Input: dimensioned drawing with shaded views. Units: mm. Origin: part minimum x, y, z. Give positions to 0.01 mm unless a question says otherwise; leave off trailing zeros. Write each loop counter-clockwise with the first axis right and the second up, starting at its lowest first coordinate (ties: lowest second). Pieces come first, ordered by that corner, then holes.
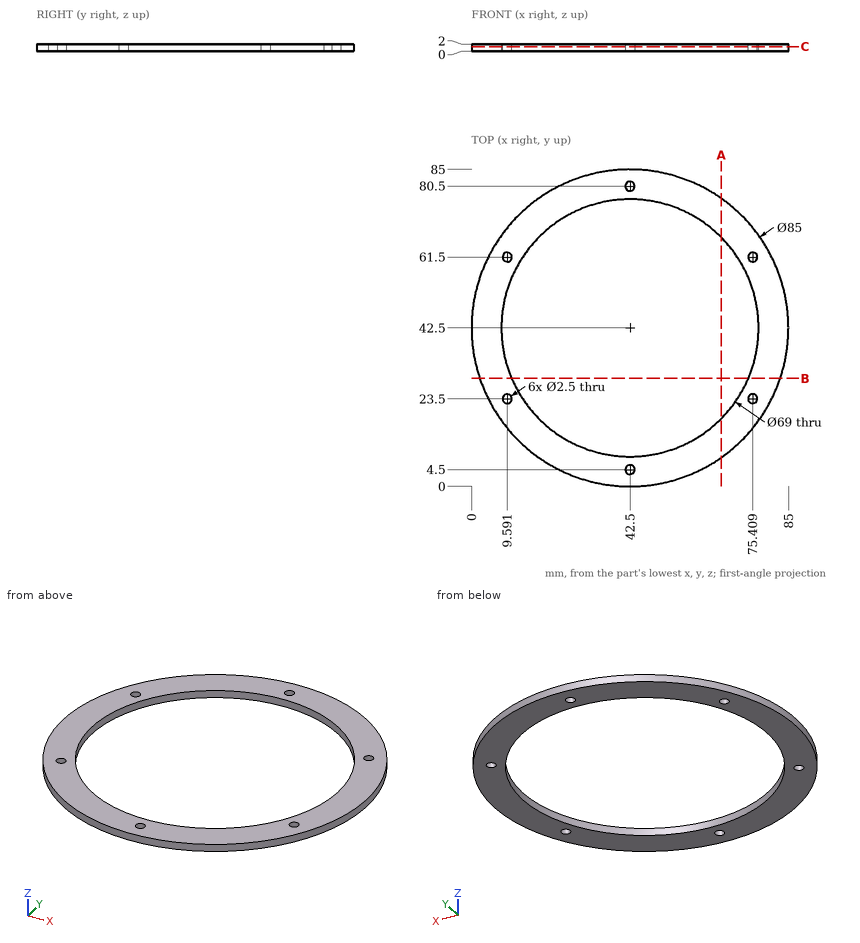
Item 1: Line query: L1, parallel to X at y = 61, z = 1.85; L2, parallel to X at y = 43.5, z = 1.3; L3, parallel to X at y = 48.5, z = 0.8. Output: solid intervals per line, ascending.
Found:
L1: x = 4.24 to 8.45, 10.74 to 13.38, 71.62 to 74.26, 76.55 to 80.76
L2: x = 0.01 to 8.01, 76.99 to 84.99
L3: x = 0.43 to 8.53, 76.47 to 84.57
Item 2: Section C-C, the plane z = 1.3. Return the cut outline in (x, y).
Found:
outline: circle Ø85 at (42.5, 42.5); hole circle Ø69 at (42.5, 42.5); hole circle Ø2.5 at (9.59, 23.5); hole circle Ø2.5 at (9.59, 61.5); hole circle Ø2.5 at (42.5, 4.5); hole circle Ø2.5 at (42.5, 80.5); hole circle Ø2.5 at (75.41, 23.5); hole circle Ø2.5 at (75.41, 61.5)
Item 3: Section A-A, the plane x = 67. Return the cut outline in (y, z).
Found:
outline: (7.77, 0) - (18.21, 0) - (18.21, 2) - (7.77, 2) - close; (66.79, 0) - (77.23, 0) - (77.23, 2) - (66.79, 2) - close
Item 4: Pin query (flat end, axial travel): pin 1 Ø3 at (x, y) = (42.5, 4.5) entering from -Z; pin 2 Ø1 at (y, z) = (11.5, 2) entering from +X. Return the tip coordinate at first contact, or that it passes through.
Found:
pin 1: stops at z = 0
pin 2: stops at x = 72.1
Item 5: Section B-B, the plane y = 29. Return the cut outline in (x, z).
Found:
outline: (2.2, 0) - (10.75, 0) - (10.75, 2) - (2.2, 2) - close; (74.25, 0) - (82.8, 0) - (82.8, 2) - (74.25, 2) - close
